```python
from build123d import *

# Parameters (mm, degrees)
BOSS_EXTRUDE2_DEPTH = 5.08


with BuildPart() as part:
    # Sketch1 → Boss-Extrude2 (new body)
    with BuildSketch(Plane.XY):
        Polygon((0, 0), (38.1, 0), (38.1, 38.1), (114.3, 38.1), (114.3, 50.8), (0, 50.8), align=None)
        with BuildLine():
            Line((7.9375, 6.35), (7.9375, 31.75))
            ThreePointArc((7.9375, 31.75), (9.525, 33.3375), (11.1125, 31.75))
            Line((11.1125, 31.75), (11.1125, 6.35))
            ThreePointArc((11.1125, 6.35), (9.525, 4.7625), (7.9375, 6.35))
        make_face(mode=Mode.SUBTRACT)
        with BuildLine():
            Line((30.1625, 31.75), (30.1625, 6.35))
            ThreePointArc((30.1625, 6.35), (28.575, 4.7625), (26.9875, 6.35))
            Line((26.9875, 6.35), (26.9875, 31.75))
            ThreePointArc((26.9875, 31.75), (28.575, 33.3375), (30.1625, 31.75))
        make_face(mode=Mode.SUBTRACT)
        with BuildLine():
            Line((107.95, 42.8625), (44.45, 42.8625))
            ThreePointArc((44.45, 42.8625), (42.8625, 44.45), (44.45, 46.0375))
            Line((44.45, 46.0375), (107.95, 46.0375))
            ThreePointArc((107.95, 46.0375), (109.5375, 44.45), (107.95, 42.8625))
        make_face(mode=Mode.SUBTRACT)
    extrude(amount=BOSS_EXTRUDE2_DEPTH)


solid = part.part
```
Geometry check sheet. Reference: the model listing, model coordinates, mm. A direction names the side the tool comes from. Round coordinates to 2 decimals unless told otherwise and drop trailing zeros. Order: outer loops, then holes, each group sorted by start corner. A loop starts at its lowest first (then second) coordinate and runs counter-clockwise, first axis right, second up. Notation, with made-up numbers: (23.5, -34) - (44.5, -34) arc R21 cw to (44.5, -11) - close; hole circle Ø2 at (66.25, -9). An arc over 180 degrees is marked (long way). Use a Markdown table: item, result. Add a question column.
(1) Sectioned sample at A-A, the plane x = 60.5. Enter the section's corners in (y, z).
(2) Release check for a two-part mould opening along Y. For faces 1 (the flat face through (0, 26, 3)), 2 (the flat face through (58, 50.8, 3)), 3 (the flat face through (11.112, 19, 3)) record: pulls with the +Y half, pulls with the -Y half, needs draft (parallel to the pull), parting line crosses it, or undercut.
(3) Sectioned sample at C-C, the plane y = 22. Enter the section's corners in (x, z).
(4) Material ranges on line 1 along X through (y, z) = (12.5, 4.5); line 2 along X through (y, z) = (32, 2.25); line 3 along Y through (x, z) = (92, 0.75), recorded low to high. Write a range as [from, to].
(5) Sectioned sample at B-B, the plane y = 44.45. Enter the section's corners in (x, z), and give its area (3 significant figures).
(6) Depth check by flat-ended pin: pin 1 (2 mm diameter, centred on x = 67.5, z = 4.5, fed in from -Y); pin 2 (3 mm diameter, centred on x = 15.5, z = 3.5, fed in from -Y); pin 3 (1.5 mm diameter, centred on y = 10, z = 1.5, fed in from +X). Enter the tip coordinate at first touch or a pass-through.
(7) Tool access check on faces 4 (the flat face through (31, 31, 5.08)), 5 (the cylindrical face through (109.537, 44.485, 2.504)), 6 (the flat face through (76, 38.1, 3)). Record the directions out of +Z, -Z, +X, -X, +Y, -Y that give a thin tool (end or side, any length) a straight path to the whole face; none if there is none.
(8) Sectioned sample at D-D, the plane z = 2.35. Count the separate pieces of the cut face and the enclosed holes in it, and give its area (3 significant figures).
Answers below:
| question | item | result |
|---|---|---|
| 1 | outline | (38.1, 0) - (42.86, 0) - (42.86, 5.08) - (38.1, 5.08) - close; (46.04, 0) - (50.8, 0) - (50.8, 5.08) - (46.04, 5.08) - close |
| 2 | face 1 | needs draft |
| 2 | face 2 | pulls with the +Y half |
| 2 | face 3 | undercut |
| 3 | outline | (0, 0) - (7.94, 0) - (7.94, 5.08) - (0, 5.08) - close; (11.11, 0) - (26.99, 0) - (26.99, 5.08) - (11.11, 5.08) - close; (30.16, 0) - (38.1, 0) - (38.1, 5.08) - (30.16, 5.08) - close |
| 4 | line 1 | [0, 7.94], [11.11, 26.99], [30.16, 38.1] |
| 4 | line 2 | [0, 7.96], [11.09, 27.01], [30.14, 38.1] |
| 4 | line 3 | [38.1, 42.86], [46.04, 50.8] |
| 5 | outline | (0, 0) - (42.86, 0) - (42.86, 5.08) - (0, 5.08) - close; (109.54, 0) - (114.3, 0) - (114.3, 5.08) - (109.54, 5.08) - close |
| 5 | area | 242 mm² |
| 6 | pin 1 | y = 38.1 |
| 6 | pin 2 | y = 0 |
| 6 | pin 3 | x = 38.1 |
| 7 | face 4 | +Z, +X, -X, +Y, -Y |
| 7 | face 5 | +Z, -Z |
| 7 | face 6 | +Z, -Z, +X, -Y |
| 8 | separate pieces | 1 |
| 8 | enclosed holes | 3 |
| 8 | area | 2,520 mm² |
